Study the drawing (mm; zero at the part's minimum x, y, z) and answer. Round coordinates to 2 decimals unless told otherwise and drop trailing zeros. Loops run counter-clockwise (first coordinate to the right, second up) from the corner with the lowest first, then second, coordinate; pieces in that order, holes last. Notation, with made-up numbers: (37, 22.25) -> (64, 22.25) arc R9 cw to (64, 26.25) -> close; hole circle Ø9 at (44.25, 72.25). An arc over 180 degrees is marked (long way). Use one line per item in the form item = value.
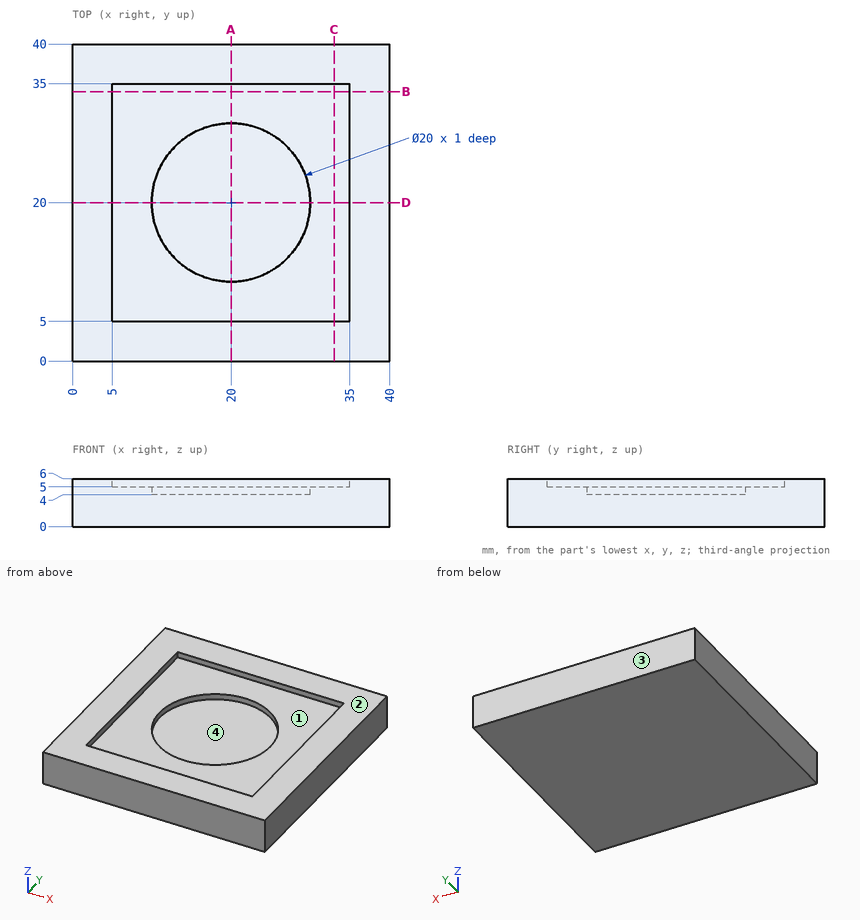
(1) Find section B-B, the plane y = 34. Write down the section's boundary in (x, z), then the cut area to 3 significant figures.
Completed:
outline = (0, 0) -> (40, 0) -> (40, 6) -> (35, 6) -> (35, 5) -> (5, 5) -> (5, 6) -> (0, 6) -> close
area = 210 mm2
(2) For a pull along Y with two mould halves and no side action, classify the marked faces 1, 2, 3 and 4 as +Y half, -Y half, draft (parallel to the pull), parting line (faces both ways), or undercut.
Completed:
face_1 = undercut
face_2 = draft
face_3 = +Y half
face_4 = undercut
(3) Find section A-A, the plane x = 20. Write down the section's boundary in (y, z).
Completed:
outline = (0, 0) -> (40, 0) -> (40, 6) -> (35, 6) -> (35, 5) -> (30, 5) -> (30, 4) -> (10, 4) -> (10, 5) -> (5, 5) -> (5, 6) -> (0, 6) -> close
(4) Given P1, Ø6, axis at x = 23, y = 20.5, coming from the +Z side, flat-ended and moving along its own axis, determine where the tip first touches the part or whether it passes through.
Completed:
P1 = 4
(5) Consider L1, parallel to Y at x = 20, z = 4.4; L2, parallel to X at y = 31, z = 5.2. Determine where each line is inside the solid, lowest interval first.
Completed:
L1 = 0 to 10, 30 to 40
L2 = 0 to 5, 35 to 40
